For this review, take the finished solid that the model builds, in its own axes (mm). Face numbers are marked on the shaded views. A direction names the side the tool comes from. Give positions to 0.01 mm unless a question says otherwise; leave off trailing zeros. Loops run counter-clockwise (first coordinate to the right, second up) from the corner with the lowest first, then second, coordinate; pieces in that order, holes last. Notation, with made-up numbers: (-12.5, 38) -> (26.5, 38) arc R24 ccw to (26.5, 49) -> close; hole circle Ø1 at (74, 58.5). An arc over 180 degrees is marked (long way). Answer as CSV lines item,"result". Start each with the question number.
Item 1: Machinability: for the marked faces 4, 5, 6, 7 and 8, which of the approach directions +Z, -Z, +X, -X, +Y, -Y give a long, thin tool a straight path to every point of the face, cutting with its end or side? Answer none if there is none.
Item 2: Add section D-D on z = 14.5. State the section outline as (x, y) points.
Item 3: The part is to be moulded in two halves that separate along X. For the marked faces 1, 2 and 3, say which applies: +X half, -X half, draft (parallel to the pull), parting line (faces both ways), or undercut.
Item 4: Add section C-C on x = 1.5. State the section outline as (y, z) points, plus the area to 3 significant figures.
Item 5: Add section A-A on z = 5.5. State the section outline as (x, y) points (3 decimals).
Item 6: Add section B-B on y = -14.75. State the section outline as (x, z) points (3 decimals), plus the area to 3 significant figures.
Item 7: For L1, parallel to Y at x = -9, z = 0.4; L2, parallel to X at y = -4.25, z = 0.3 (3 decimals); L3, parallel to X at y = -3.75, z = 5.75 (3 decimals), list the stretches that pass through material, from the lowest coordinate up. Write a range as from..to.
Item 8: Clearance check with flat-ended pins moving along their axes: P1, Ø8, axis at y = -2.5, z = 12.5, coming from the -X side; P2, Ø1.5, axis at x = 11, y = -5, coming from the +Z side; P3, Ø4, axis at x = 5.5, y = -5, coming from the +Z side. State where each tip first meets the part, or that it passes through.
```python
from build123d import *

# Parameters (mm, degrees)
PAD015_DEPTH         = 17.3
POCKET009_DEPTH      = 0.001
POCKET009_DEPTH_BACK = 11.501
SKETCH022_R          = 1.4
POCKET007_DEPTH      = 0.001
POCKET007_DEPTH_BACK = 11.501
POCKET008_DEPTH      = 2
POCKET008_DEPTH_BACK = 1
SKETCH026_W          = 18
SKETCH026_H          = 2.75
POCKET006_DEPTH      = 4
SKETCH027_W          = 12.25
SKETCH027_H          = 1.5
SKETCH027_H_2        = 2
POCKET010_DEPTH      = 10
PAD016_DEPTH         = 6.5


with BuildPart() as part:
    # Sketch024 → Pad015 (new body)
    with BuildSketch(Plane.XZ):
        with BuildLine():
            Line((-13.5, 0), (-6.125, 0))
            Line((-6.125, 0), (-6.125, 7.5))
            ThreePointArc((-3.625, 10), (-5.392767, 9.267767), (-6.125, 7.5))
            Line((-3.625, 10), (3.625, 10))
            ThreePointArc((6.125, 7.5), (5.392767, 9.267767), (3.625, 10))
            Line((6.125, 7.5), (6.125, 0))
            Line((6.125, 0), (13.5, 0))
            Line((13.5, 0), (13.5, 3))
            Line((13.5, 3), (8.5, 3))
            ThreePointArc((7.5, 4), (7.792893, 3.292893), (8.5, 3))
            Line((7.5, 4), (7.5, 10.5))
            ThreePointArc((7.5, 10.5), (7.207107, 11.207107), (6.5, 11.5))
            Line((6.5, 11.5), (-6.5, 11.5))
            ThreePointArc((-6.5, 11.5), (-7.207107, 11.207107), (-7.5, 10.5))
            Line((-7.5, 10.5), (-7.5, 4))
            ThreePointArc((-8.5, 3), (-7.792893, 3.292893), (-7.5, 4))
            Line((-8.5, 3), (-13.5, 3))
            Line((-13.5, 3), (-13.5, 0))
        make_face()
    extrude(amount=PAD015_DEPTH)

    # Sketch023 → Pocket009 (cut, two sides)
    with BuildSketch(Plane.XY) as pocket009_sk:
        with BuildLine():
            Line((-9.375, 0), (9.375, 0))
            ThreePointArc((13.375, -4), (12.203427, -1.171573), (9.375, 0))
            Line((13.375, -4), (13.375, -4.5))
            ThreePointArc((9.375, -8.5), (12.203427, -7.328427), (13.375, -4.5))
            Line((9.375, -8.5), (7.5, -8.5))
            Line((7.5, -8.5), (7.5, -29))
            Line((7.5, -29), (15, -29))
            Line((15, -29), (15, 1))
            Line((15, 1), (-15, 1))
            Line((-15, 1), (-15, -29))
            Line((-15, -29), (-7.5, -29))
            Line((-7.5, -29), (-7.5, -8.5))
            Line((-7.5, -8.5), (-9.375, -8.5))
            ThreePointArc((-13.375, -4.5), (-12.203427, -7.328427), (-9.375, -8.5))
            Line((-13.375, -4.5), (-13.375, -4))
            ThreePointArc((-9.375, 0), (-12.203427, -1.171573), (-13.375, -4))
        make_face()
    extrude(amount=-POCKET009_DEPTH, mode=Mode.SUBTRACT)
    extrude(pocket009_sk.sketch, amount=POCKET009_DEPTH_BACK, mode=Mode.SUBTRACT)

    # Sketch022 → Pocket007 (cut, two sides)
    with BuildSketch(Plane.XY) as pocket007_sk:
        with Locations((-9, -4.25)):
            Circle(SKETCH022_R)
        with Locations((9, -4.25)):
            Circle(SKETCH022_R)
    extrude(amount=-POCKET007_DEPTH, mode=Mode.SUBTRACT)
    extrude(pocket007_sk.sketch, amount=POCKET007_DEPTH_BACK, mode=Mode.SUBTRACT)

    # Sketch025 (on DatumPlane) → Pocket008 (cut, two sides)
    with BuildSketch(Plane.XY.offset(3)) as pocket008_sk:
        Polygon((-6.375, -5.765544), (-6.375, -2.734456), (-9, -1.218911), (-11.625, -2.734456), (-11.625, -5.765544), (-9, -7.281089), align=None)
        Polygon((11.625, -5.765544), (11.625, -2.734456), (9, -1.218911), (6.375, -2.734456), (6.375, -5.765544), (9, -7.281089), align=None)
    extrude(amount=-POCKET008_DEPTH, mode=Mode.SUBTRACT)
    extrude(pocket008_sk.sketch, amount=POCKET008_DEPTH_BACK, mode=Mode.SUBTRACT)

    # Sketch026 → Pocket006 (cut)
    with BuildSketch(Plane.XY):
        with Locations((0, -4.25)):
            Rectangle(SKETCH026_W, SKETCH026_H)
    extrude(amount=POCKET006_DEPTH, mode=Mode.SUBTRACT)

    # Sketch027 → Pocket010 (cut)
    with BuildSketch(Plane.XY):
        with Locations((0, -8.5)):
            Rectangle(SKETCH027_W, SKETCH027_H)
        with Locations((0, -11.5)):
            Rectangle(SKETCH027_W, SKETCH027_H)
        with Locations((0, -16.75)):
            Rectangle(SKETCH027_W, SKETCH027_H_2)
    extrude(amount=POCKET010_DEPTH, mode=Mode.SUBTRACT)

    # Sketch028 → Pad016 (join, symmetric)
    with BuildSketch(Plane.YZ):
        with BuildLine():
            Line((-13, 11.5), (-8, 11.5))
            Line((-11.566987, 17.678203), (-8, 11.5))
            ThreePointArc((-11.566987, 17.678203), (-12.109054, 17.916166), (-12.498243, 17.470078))
            Line((-13, 11.5), (-12.498243, 17.470078))
        make_face()
    extrude(amount=PAD016_DEPTH, both=True)


solid = part.part
```
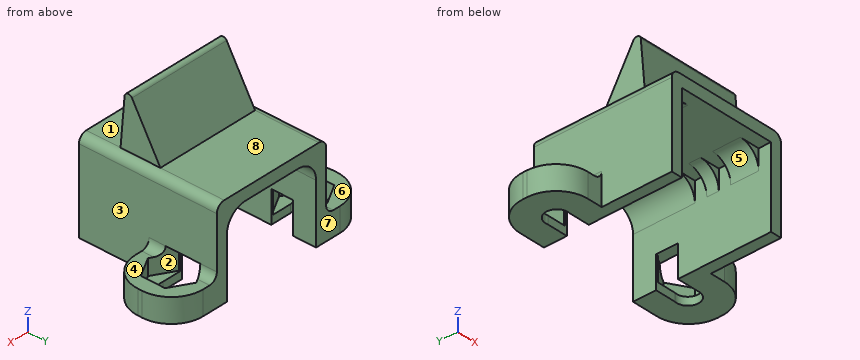
Computed values:
1,face 4,"+Z, +X, +Y, -Y"
1,face 5,"-Z, +Y, -Y"
1,face 6,"+Z, -X, +Y, -Y"
1,face 7,"+Z, -Z, +X, -X, +Y"
1,face 8,"+Z, +X, -X, +Y"
2,outline,"(-6.5, -12.75) -> (6.5, -12.75) -> (6.5, -9.73) -> (-6.5, -9.73) -> close"
3,face 1,"draft"
3,face 2,"undercut"
3,face 3,"+X half"
4,outline,"(-17.3, 10) -> (0, 10) -> (0, 11.5) -> (-8, 11.5) -> (-11.57, 17.68) arc R0.5 ccw to (-12.5, 17.47) -> (-13, 11.5) -> (-17.3, 11.5) -> close"
4,area,"44.4 mm²"
5,outline,"(-7.5, -17.3) -> (-6.125, -17.3) -> (-6.125, 0) -> (-7.5, 0) -> close; (6.125, -17.3) -> (7.5, -17.3) -> (7.5, 0) -> (6.125, 0) -> close"
6,outline,"(-7.5, 0) -> (-6.125, 0) -> (-6.125, 7.5) arc R2.5 cw to (-3.625, 10) -> (3.625, 10) arc R2.5 cw to (6.125, 7.5) -> (6.125, 0) -> (7.5, 0) -> (7.5, 10.5) arc R1 ccw to (6.5, 11.5) -> (-6.5, 11.5) arc R1 ccw to (-7.5, 10.5) -> close"
6,area,"52.3 mm²"
7,L1,"-8.5..-5.65, -2.85..0"
7,L2,"-13.375..-10.4, 10.4..13.375"
7,L3,"-7.5..-6.125, 6.125..7.5"
8,P1,"x = -7.5"
8,P2,"z = 3"
8,P3,"z = 11.5"
